from build123d import *

# Parameters (mm, degrees)
SKETCH1_W            = 8.382
SKETCH1_H            = 13.3858
BOSS_EXTRUDE1_DEPTH  = 7.366
SKETCH2_W            = 5.588
SKETCH2_H            = 0.635
BOSS_EXTRUDE2_DEPTH  = 0.635
SKETCH3_W            = 5.588
SKETCH3_H            = 0.635
BOSS_EXTRUDE3_DEPTH  = 0.635
SKETCH4_W            = 0.635
SKETCH4_H            = 0.635
BOSS_EXTRUDE4_DEPTH  = 5.207
SKETCH5_W            = 0.635
SKETCH5_H            = 0.635
BOSS_EXTRUDE5_DEPTH  = 5.207
SKETCH6_W            = 0.635
SKETCH6_H            = 0.635
BOSS_EXTRUDE6_DEPTH  = 5.207
SKETCH7_W            = 0.635
SKETCH7_H            = 0.635
BOSS_EXTRUDE7_DEPTH  = 5.207
SKETCH8_W            = 0.635
SKETCH8_H            = 0.635
BOSS_EXTRUDE8_DEPTH  = 5.207
SKETCH9_W            = 0.635
SKETCH9_H            = 0.635
BOSS_EXTRUDE9_DEPTH  = 5.207
SKETCH10_W           = 0.635
SKETCH10_H           = 0.635
BOSS_EXTRUDE10_DEPTH = 5.207
SKETCH11_W           = 0.635
SKETCH11_H           = 0.635
BOSS_EXTRUDE11_DEPTH = 5.207
SKETCH12_W           = 0.635
SKETCH12_H           = 0.635
BOSS_EXTRUDE12_DEPTH = 5.207
SKETCH13_W           = 0.635
SKETCH13_H           = 0.635
BOSS_EXTRUDE13_DEPTH = 5.207
SKETCH14_W           = 0.762
SKETCH14_H           = 5.588
CUT_EXTRUDE1_DEPTH   = 0.999998
SKETCH15_W           = 0.762
SKETCH15_H           = 5.588
CUT_EXTRUDE2_DEPTH   = 0.999998
FILLET1_R            = 0.8128


with BuildPart() as part:
    # Sketch1 → Boss-Extrude1 (new body)
    with BuildSketch(Plane(origin=(-3.683, 0, 0), x_dir=(0, -1, 0), z_dir=(-1, 0, 0))):
        with Locations((0.381, -6.6929)):
            Rectangle(SKETCH1_W, SKETCH1_H)
    extrude(amount=-BOSS_EXTRUDE1_DEPTH)

    # Sketch2 → Boss-Extrude2 (add)
    with BuildSketch(Plane.XZ.offset(4.572)):
        with Locations((0, -2.8829)):
            Rectangle(SKETCH2_W, SKETCH2_H)
    extrude(amount=BOSS_EXTRUDE2_DEPTH)

    # Sketch3 → Boss-Extrude3 (add)
    with BuildSketch(Plane.XZ.offset(4.572)):
        with Locations((0, -10.5029)):
            Rectangle(SKETCH3_W, SKETCH3_H)
    extrude(amount=BOSS_EXTRUDE3_DEPTH)

    # Sketch4 → Boss-Extrude4 (add)
    with BuildSketch(Plane.XZ.offset(4.572)):
        with Locations((1.27, -11.7729)):
            Rectangle(SKETCH4_W, SKETCH4_H)
    extrude(amount=BOSS_EXTRUDE4_DEPTH)

    # Sketch5 → Boss-Extrude5 (add)
    with BuildSketch(Plane.XZ.offset(4.572)):
        with Locations((-1.27, -11.7729)):
            Rectangle(SKETCH5_W, SKETCH5_H)
    extrude(amount=BOSS_EXTRUDE5_DEPTH)

    # Sketch6 → Boss-Extrude6 (add)
    with BuildSketch(Plane.XZ.offset(4.572)):
        with Locations((1.27, -9.2329)):
            Rectangle(SKETCH6_W, SKETCH6_H)
    extrude(amount=BOSS_EXTRUDE6_DEPTH)

    # Sketch7 → Boss-Extrude7 (add)
    with BuildSketch(Plane.XZ.offset(4.572)):
        with Locations((-1.27, -9.2329)):
            Rectangle(SKETCH7_W, SKETCH7_H)
    extrude(amount=BOSS_EXTRUDE7_DEPTH)

    # Sketch8 → Boss-Extrude8 (add)
    with BuildSketch(Plane.XZ.offset(4.572)):
        with Locations((1.27, -6.6929)):
            Rectangle(SKETCH8_W, SKETCH8_H)
    extrude(amount=BOSS_EXTRUDE8_DEPTH)

    # Sketch9 → Boss-Extrude9 (add)
    with BuildSketch(Plane.XZ.offset(4.572)):
        with Locations((-1.27, -6.6929)):
            Rectangle(SKETCH9_W, SKETCH9_H)
    extrude(amount=BOSS_EXTRUDE9_DEPTH)

    # Sketch10 → Boss-Extrude10 (add)
    with BuildSketch(Plane.XZ.offset(4.572)):
        with Locations((1.27, -4.1529)):
            Rectangle(SKETCH10_W, SKETCH10_H)
    extrude(amount=BOSS_EXTRUDE10_DEPTH)

    # Sketch11 → Boss-Extrude11 (add)
    with BuildSketch(Plane.XZ.offset(4.572)):
        with Locations((-1.27, -4.1529)):
            Rectangle(SKETCH11_W, SKETCH11_H)
    extrude(amount=BOSS_EXTRUDE11_DEPTH)

    # Sketch12 → Boss-Extrude12 (add)
    with BuildSketch(Plane.XZ.offset(4.572)):
        with Locations((1.27, -1.6129)):
            Rectangle(SKETCH12_W, SKETCH12_H)
    extrude(amount=BOSS_EXTRUDE12_DEPTH)

    # Sketch13 → Boss-Extrude13 (add)
    with BuildSketch(Plane.XZ.offset(4.572)):
        with Locations((-1.27, -1.6129)):
            Rectangle(SKETCH13_W, SKETCH13_H)
    extrude(amount=BOSS_EXTRUDE13_DEPTH)

    # Sketch14 → Cut-Extrude1 (cut)
    with BuildSketch(Plane(origin=(0, 3.81, 0), x_dir=(-1, 0, 0), z_dir=(0, 1, 0))):
        with Locations((2.794, -6.6929)):
            Rectangle(SKETCH14_W, SKETCH14_H)
    extrude(amount=-CUT_EXTRUDE1_DEPTH, mode=Mode.SUBTRACT)

    # Sketch15 → Cut-Extrude2 (cut)
    with BuildSketch(Plane(origin=(0, 3.81, 0), x_dir=(-1, 0, 0), z_dir=(0, 1, 0))):
        with Locations((-2.794, -6.6929)):
            Rectangle(SKETCH15_W, SKETCH15_H)
    extrude(amount=-CUT_EXTRUDE2_DEPTH, mode=Mode.SUBTRACT)

    # Sketch16 → Hole1 (revolve, cut)
    with BuildSketch(Plane(origin=(0, 0, 0), x_dir=(0, -1, 0), z_dir=(1, 0, 0))):
        Polygon((0, 0), (0, 2.0574), (1.8034, 2.0574), (1.8034, 1.0414), (2.8448, 0), align=None)
    revolve(axis=Axis((0, 0, 6.445314094), (0, 0, -1)), mode=Mode.SUBTRACT)

    # Sketch18 → Hole2 (revolve, cut)
    with BuildSketch(Plane(origin=(0, 0, -13.3858), x_dir=(0, 1, 0), z_dir=(1, 0, 0))):
        Polygon((0, 0), (0, 2.0574), (1.8034, 2.0574), (1.8034, 1.0414), (2.8448, 0), align=None)
    revolve(axis=Axis((0, 0, -19.831114094), (0, 0, 1)), mode=Mode.SUBTRACT)

    # Fillet1
    # the kernel refuses this fillet: 0.8128 mm, written as the material it takes off along each edge
    with BuildSketch(Plane(origin=(-2.8702, 2.9972, -12.573), x_dir=(-1, 0, 0), z_dir=(0, 0, -1))) as fillet1_piece_1_section:
        Polygon((0, 0), (FILLET1_R, 0), (FILLET1_R, FILLET1_R), (0, FILLET1_R), align=None)
    fillet1_piece_1 = extrude(amount=FILLET1_R, mode=Mode.PRIVATE)
    fillet1_piece_1 = fillet1_piece_1 - Plane(origin=(-2.8702, 2.9972, -12.573), x_dir=(0.7071067811865475, -0.7071067811865475, 0), z_dir=(0, 0, -1)) * Sphere(FILLET1_R, mode=Mode.PRIVATE)
    add(fillet1_piece_1, mode=Mode.SUBTRACT)
    with BuildSketch(Plane(origin=(2.8702, 2.9972, -12.573), x_dir=(1, 0, 0), z_dir=(0, 0, -1))) as fillet1_piece_2_section:
        Polygon((0, 0), (FILLET1_R, 0), (FILLET1_R, -FILLET1_R), (0, -FILLET1_R), align=None)
    fillet1_piece_2 = extrude(amount=FILLET1_R, mode=Mode.PRIVATE)
    fillet1_piece_2 = fillet1_piece_2 - Plane(origin=(2.8702, 2.9972, -12.573), x_dir=(-0.7071067811865475, -0.7071067811865475, 0), z_dir=(0, 0, -1)) * Sphere(FILLET1_R, mode=Mode.PRIVATE)
    add(fillet1_piece_2, mode=Mode.SUBTRACT)
    with BuildSketch(Plane(origin=(-2.8702, 2.9972, -0.8128), x_dir=(0, 0, 1), z_dir=(-1, 0, 0))) as fillet1_piece_3_section:
        Polygon((0, 0), (FILLET1_R, 0), (FILLET1_R, FILLET1_R), (0, FILLET1_R), align=None)
    fillet1_piece_3 = extrude(amount=FILLET1_R, mode=Mode.PRIVATE)
    fillet1_piece_3 = fillet1_piece_3 - Plane(origin=(-2.8702, 2.9972, -0.8128), x_dir=(0, -0.7071067811865475, -0.7071067811865475), z_dir=(-1, 0, 0)) * Sphere(FILLET1_R, mode=Mode.PRIVATE)
    add(fillet1_piece_3, mode=Mode.SUBTRACT)
    with BuildSketch(Plane(origin=(2.8702, 2.9972, -0.8128), x_dir=(0, 0, 1), z_dir=(1, 0, 0))) as fillet1_piece_4_section:
        Polygon((0, 0), (FILLET1_R, 0), (FILLET1_R, -FILLET1_R), (0, -FILLET1_R), align=None)
    fillet1_piece_4 = extrude(amount=FILLET1_R, mode=Mode.PRIVATE)
    fillet1_piece_4 = fillet1_piece_4 - Plane(origin=(2.8702, 2.9972, -0.8128), x_dir=(0, -0.7071067811865475, -0.7071067811865475), z_dir=(1, 0, 0)) * Sphere(FILLET1_R, mode=Mode.PRIVATE)
    add(fillet1_piece_4, mode=Mode.SUBTRACT)
    with BuildSketch(Plane(origin=(-3.683, 2.9972, -13.3858), x_dir=(1, 0, 0), z_dir=(0, -1, 0)), Plane(origin=(3.683, -6.604, 0), x_dir=(0, 0, -1), z_dir=(0, 1, 0))) as fillet1_piece_5:
        with BuildLine():
            CenterArc((FILLET1_R, FILLET1_R), FILLET1_R, 180, 90)
            Line((0, FILLET1_R), (0, 0))
            Line((0, 0), (FILLET1_R, 0))
        make_face()
    extrude(amount=9.6012, mode=Mode.SUBTRACT)
    with BuildSketch(Plane(origin=(-2.8702, 3.81, -13.3858), x_dir=(0, -1, 0), z_dir=(1, 0, 0))) as fillet1_piece_6:
        with BuildLine():
            CenterArc((FILLET1_R, -FILLET1_R), FILLET1_R, 90, 90)
            Line((0, -FILLET1_R), (0, 0))
            Line((0, 0), (FILLET1_R, 0))
        make_face()
    extrude(amount=5.7404, mode=Mode.SUBTRACT)
    with BuildSketch(Plane(origin=(3.683, 2.9972, -13.3858), x_dir=(-1, 0, 0), z_dir=(0, -1, 0)), Plane(origin=(-3.683, -6.604, 0), x_dir=(0, 0, -1), z_dir=(0, 1, 0))) as fillet1_piece_7:
        with BuildLine():
            CenterArc((FILLET1_R, -FILLET1_R), FILLET1_R, 90, 90)
            Line((0, -FILLET1_R), (0, 0))
            Line((0, 0), (FILLET1_R, 0))
        make_face()
    extrude(amount=9.6012, mode=Mode.SUBTRACT)
    with BuildSketch(Plane(origin=(-3.683, 3.81, -0.8128), x_dir=(0, -1, 0), z_dir=(0, 0, -1))) as fillet1_piece_8:
        with BuildLine():
            CenterArc((FILLET1_R, -FILLET1_R), FILLET1_R, 90, 90)
            Line((0, -FILLET1_R), (0, 0))
            Line((0, 0), (FILLET1_R, 0))
        make_face()
    extrude(amount=11.7602, mode=Mode.SUBTRACT)
    with BuildSketch(Plane(origin=(3.683, 3.81, -0.8128), x_dir=(0, -1, 0), z_dir=(0, 0, -1))) as fillet1_piece_9:
        with BuildLine():
            CenterArc((FILLET1_R, FILLET1_R), FILLET1_R, 180, 90)
            Line((0, FILLET1_R), (0, 0))
            Line((0, 0), (FILLET1_R, 0))
        make_face()
    extrude(amount=11.7602, mode=Mode.SUBTRACT)
    with BuildSketch(Plane(origin=(-2.8702, 3.81, 0), x_dir=(0, -1, 0), z_dir=(1, 0, 0))) as fillet1_piece_10:
        with BuildLine():
            CenterArc((FILLET1_R, FILLET1_R), FILLET1_R, 180, 90)
            Line((0, FILLET1_R), (0, 0))
            Line((0, 0), (FILLET1_R, 0))
        make_face()
    extrude(amount=5.7404, mode=Mode.SUBTRACT)


solid = part.part
Read the model definition and answer for the solid it produces. Units are mm, in the model's axes. A direction names the side the tool comes from. Round coordinates to 2 decimals unless told otherwise and drop trailing zeros. Write each loop counter-clockwise with the first axis right and the second up, starting at its lowest first coordinate (ties: lowest second). Pieces come first, ordered by that corner, then holes. Notation, with made-up numbers: (40.25, 15) - (77.25, 15) arc R8 cw to (77.25, 28) - close; hole circle Ø10 at (45.5, 21). An arc over 180 degrees is marked (long way). One line per question, with ' | ' between items. Start each with the question number.
1. For a pull along X with two mould halves and no side action, classify faces 6 (the face through (0, -3, -13.386)), 7 (the face through (1.1, 1.43, -1.54)), 8 (the face through (-3.45, -0.73, -13.14)) as +X half, -X half, draft (parallel to the pull), parting line (faces both ways), or undercut.
2. Section C-C (z = -4.75) is taken. Determine the outline of the cut face in (x, y) (3 decimals).
3. Find the intervals of material crossed by probe 1 along Z at (x, y) = (1, -7); probe 2 along X at (y, z) = (0, -1.3); probe 3 along Y at (x, z) = (0, -11.65), in increasing order. Write a range as [from, to].
4. For faces 1 (the face through (-0.04, 3.57, -13.15)), 2 (the face through (0, -3, 0)), 3 (the face through (0, 0, -11.328)), 4 (the face through (0, 0, -2.057)), 5 (the face through (3.175, 3, -7)), determine the directions among +Z, -Z, +X, -X, +Y, -Y from which every point of the face is accessible in a straight line to the end or side of a thin tool.
5. Each of these flat-tipped pins is pushed along its axis until it touches: pin 1 (2 mm diameter, centred on x = -2.5, y = 1, fed in from -Z); pin 2 (0.5 mm diameter, centred on y = -6, z = -4, fed in from -X); pin 3 (0.6 mm diameter, centred on x = 3, z = -7, fed in from +Y); pin 4 (0.5 mm diameter, centred on x = -1.5, y = -7.5, fed in from +Z). Where does it stop, or does it pass through?
6. Section B-B (x = 0) is taken. Determine the outline of the cut face in (y, z).
Filled in:
1) face 6: draft | face 7: undercut | face 8: -X half
2) outline: (-3.683, -4.572) - (3.683, -4.572) - (3.683, 2.997) arc R0.813 ccw to (3.175, 3.751) - (3.175, 2.81) - (2.413, 2.81) - (2.413, 3.81) - (-2.413, 3.81) - (-2.413, 2.81) - (-3.175, 2.81) - (-3.175, 3.751) arc R0.813 ccw to (-3.683, 2.997) - close
3) probe 1: [-12.09, -11.46], [-9.55, -8.92], [-7.01, -6.38], [-4.47, -3.84], [-1.93, -1.3] | probe 2: [-3.68, -1.8], [1.8, 3.68] | probe 3: [-4.57, -1.8], [1.8, 3.81]
4) face 1: -Z, +X, -X, +Y | face 2: +Z, +X, -X, +Y, -Y | face 3: -Z | face 4: +Z | face 5: +Y
5) pin 1: z = -13.39 | pin 2: x = -1.59 | pin 3: y = 3.75 | pin 4: z = -1.3
6) outline: (-5.21, -10.82) - (-4.57, -10.82) - (-4.57, -13.39) - (-2.84, -13.39) - (-1.8, -12.34) - (-1.8, -11.33) - (1.8, -11.33) - (1.8, -12.34) - (2.84, -13.39) - (3, -13.39) arc R0.81 ccw to (3.81, -12.57) - (3.81, -0.81) arc R0.81 ccw to (3, 0) - (2.84, 0) - (1.8, -1.04) - (1.8, -2.06) - (-1.8, -2.06) - (-1.8, -1.04) - (-2.84, 0) - (-4.57, 0) - (-4.57, -2.57) - (-5.21, -2.57) - (-5.21, -3.2) - (-4.57, -3.2) - (-4.57, -10.19) - (-5.21, -10.19) - close
